Geometry: final body of the model. Coordinates: model frame, mm. A direction names the side the tool comes from. Give positions to 0.01 mm unless a question says otherwise; leave off trailing zeros. Write each loop counter-clockwise with the first axis right and the second up, starting at its lowest first coordinate (ties: lowest second). Pieces come first, ordered by that corner, then holes. Notation, with made-up numbers: M 47.5,-27.75 L 63.5,-27.75 A25 ccw 63.5,-15.75 Z; hole C 84.5,39.25 d4. An arc over 180 degrees is marked long. Use a Markdown table: item, result. Add a question column.
1) Line query: line 1 (Y direction, x = -46.5, z = 1.15); line 2 (X direction, y = -2, z = 1.7); line 3 (Y direction, x = -55, z = 1.5). Output: solid intervals per line, ascending.
2) Set-up query: faces 1 (the flat face through (-42, -6.5, 1)), 2 (the flat face through (-1, 9.5, 1)). Return all of +Z, -Z, +X, -X, +Y, -Y with unobstructed straight access to the full face (end or side cutting, diameter ignored); none if empty.
3) Section B-B on x = -6.5. Return the cut outline in (y, z).
4) Section C-C on z = 1.65. State how many separate pieces and enclosed holes the cut face has, then the cut area to 3 significant figures.
5) Draft query along X for faces 3 (the flat face through (-51, -4, 1)), 4 (the flat face through (-1, 6, 2)), 5 (the flat face through (-62, 0, 1)), 6 (the flat face through (62, 0, 1)). Return one class per face: +X half, -X half, draft (parallel to the pull), parting line (faces both ways), or undercut.
6) Section A-A on x = -40.5. Return the cut outline in (y, z).
```python
from build123d import *

# Parameters (mm, degrees)
SKETCH_1_W          = 124
SKETCH_1_H          = 19
EXTRUDE_1_DEPTH     = 2
SKETCH_3_R          = 1.6
CUT_EXTRUDE_2_DEPTH = 63.755477849
SKETCH_4_R          = 1.6
CUT_EXTRUDE_3_DEPTH = 63.755477849
SKETCH_5_W          = 56
SKETCH_5_H          = 10
CUT_EXTRUDE_4_DEPTH = 63.755477849
FILLET_1_R          = 1.3


with BuildPart() as part:
    # 草图1 → 凸台-拉伸1 (new body)
    with BuildSketch(Plane.XY):
        Rectangle(SKETCH_1_W, SKETCH_1_H)
    extrude(amount=EXTRUDE_1_DEPTH)

    # 草图3 → 切除-拉伸2 (cut, through all)
    with BuildSketch(Plane.XY.offset(2)):
        with Locations((-55, -2.5)):
            Circle(SKETCH_3_R)
        with Locations(Location((55, -2.5, 0), (0, 0, 180))):
            Circle(SKETCH_3_R)
    extrude(amount=-CUT_EXTRUDE_2_DEPTH, mode=Mode.SUBTRACT)

    # 草图4 → 切除-拉伸3 (cut, through all)
    with BuildSketch(Plane.XY.offset(2)):
        with Locations((-53.84, 6.04)):
            Circle(SKETCH_4_R)
        with Locations((-34.086233188, 2.911310699)):
            Circle(SKETCH_4_R)
        with Locations(Location((34.086233188, 2.911310699, 0), (0, 0, 180))):
            Circle(SKETCH_4_R)
        with Locations(Location((53.84, 6.04, 0), (0, 0, 180))):
            Circle(SKETCH_4_R)
    extrude(amount=-CUT_EXTRUDE_3_DEPTH, mode=Mode.SUBTRACT)

    # 草图5 → 切除-拉伸4 (cut, through all)
    with BuildSketch(Plane.XY.offset(2)):
        with BuildLine():
            Line((-49.87886563, 5.483749603), (-51, -2.5))
            Line((-51, -2.5), (-51, -6.5))
            Line((-51, -6.5), (-34.086233188, -6.5))
            Line((-34.086233188, -6.5), (-34.086233188, -1.088689301))
            ThreePointArc((-34.086233188, -1.088689301), (-37.711819735, 1.221600016), (-37.149329348, 5.483749603))
            Line((-37.149329348, 5.483749603), (-49.87886563, 5.483749603))
        make_face()
        Rectangle(SKETCH_5_W, SKETCH_5_H)
        with BuildLine():
            Line((34.086233188, -1.088689301), (34.086233188, -6.5))
            Line((34.086233188, -6.5), (51, -6.5))
            Line((51, -6.5), (51, -2.5))
            Line((51, -2.5), (49.87886563, 5.483749603))
            Line((49.87886563, 5.483749603), (37.149329348, 5.483749603))
            ThreePointArc((37.149329348, 5.483749603), (37.844715903, 4.28018165), (38.086233188, 2.911310699))
            ThreePointArc((38.086233188, 2.911310699), (36.914660313, 0.082883574), (34.086233188, -1.088689301))
        make_face()
    extrude(amount=-CUT_EXTRUDE_4_DEPTH, mode=Mode.SUBTRACT)

    # 圆角1
    fillet_1_edges = [part.edges().sort_by_distance(p)[0] for p in [
        (-37.149329348, 5.483749603, 1),
        (-34.086233188, -1.088689301, 1),
        (-51, -6.5, 1),
        (-51, -2.5, 1),
        (-49.87886563, 5.483749603, 1),
        (-28, -5, 1),
        (-28, 5, 1),
        (28, 5, 1),
        (28, -5, 1),
        (37.149329348, 5.483749603, 1),
        (49.87886563, 5.483749603, 1),
        (51, -2.5, 1),
        (51, -6.5, 1),
        (34.086233188, -6.5, 1),
        (34.086233188, -1.088689301, 1),
    ]]
    fillet(fillet_1_edges, radius=FILLET_1_R)


solid = part.part
```
Found:
| question | item | result |
|---|---|---|
| 1 | line 1 | -9.5 to -6.5, 5.48 to 9.5 |
| 1 | line 2 | -62 to -56.52, -53.48 to -50.93, -34.11 to -28, 28 to 34.11, 50.93 to 53.48, 56.52 to 62 |
| 1 | line 3 | -9.5 to -4.1, -0.9 to 4.94, 7.14 to 9.5 |
| 2 | face 1 | +Z, -Z |
| 2 | face 2 | +Z, -Z, +X, -X, +Y |
| 3 | outline | M -9.5,0 L -5,0 L -5,2 L -9.5,2 Z; M 5,0 L 9.5,0 L 9.5,2 L 5,2 Z |
| 4 | separate pieces | 1 |
| 4 | enclosed holes | 9 |
| 4 | area | 1,400 mm² |
| 5 | face 3 | undercut |
| 5 | face 4 | draft |
| 5 | face 5 | -X half |
| 5 | face 6 | +X half |
| 6 | outline | M -9.5,0 L -6.5,0 L -6.5,2 L -9.5,2 Z; M 5.48,0 L 9.5,0 L 9.5,2 L 5.48,2 Z |
